Build history of the part. All positions in model axes, mm. Face numbers are marked on the shaded views. A direction names the side the tool comes from. Coordinates: 2 decimals unless noted, no trailing zeros. Order: outer loops, then holes, each group sorted by start corner. A loop starts at its lowest first (then second) coordinate and runs counter-clockwise, first axis right, second up. Notation, with made-up numbers: (7, 33.25) -> (34, 33.25) arc R18 ccw to (34, 49.25) -> close; hole circle Ø4 at (7.25, 45.5). An arc over 180 degrees is marked (long way). Write each question's results on one line, items separated by ' | '.
from build123d import *

# Parameters (mm, degrees)
PAD003_DEPTH    = 43
SKETCH004_R     = 11.5
SKETCH004_R_2   = 1.7
POCKET_DEPTH    = 4
SKETCH005_R     = 1.8
SKETCH005_W     = 20
SKETCH005_H     = 10
POCKET001_DEPTH = 3.6
CHAMFER_SIZE    = 6


with BuildPart() as part:
    # Sketch003 → Pad003 (new body)
    with BuildSketch(Plane.XY):
        Polygon((-43, 4), (-3.6, 4), (-3.6, 24), (0, 24), (0, 0), (-43, 0), align=None)
    extrude(amount=PAD003_DEPTH)

    # Sketch004 → Pocket (cut)
    with BuildSketch(Plane.XZ):
        with Locations((-21.5, 21.5)):
            Circle(SKETCH004_R)
        with Locations((-37, 37)):
            Circle(SKETCH004_R_2)
        with Locations((-6, 37)):
            Circle(SKETCH004_R_2)
        with Locations((-6, 6)):
            Circle(SKETCH004_R_2)
        with Locations((-37, 6)):
            Circle(SKETCH004_R_2)
    extrude(amount=-POCKET_DEPTH, mode=Mode.SUBTRACT)

    # Sketch005 → Pocket001 (cut)
    with BuildSketch(Plane.YZ):
        with Locations((16, 29)):
            Circle(SKETCH005_R)
        with Locations((16, 14)):
            Circle(SKETCH005_R)
        with Locations((14, 38)):
            Rectangle(SKETCH005_W, SKETCH005_H)
        with Locations((14, 5)):
            Rectangle(SKETCH005_W, SKETCH005_H)
    extrude(amount=-POCKET001_DEPTH, mode=Mode.SUBTRACT)

    # Chamfer
    chamfer_edges = [part.edges().sort_by_distance(p)[0] for p in [
        (-3.6, 4, 21.5),
    ]]
    chamfer(chamfer_edges, length=CHAMFER_SIZE)


solid = part.part
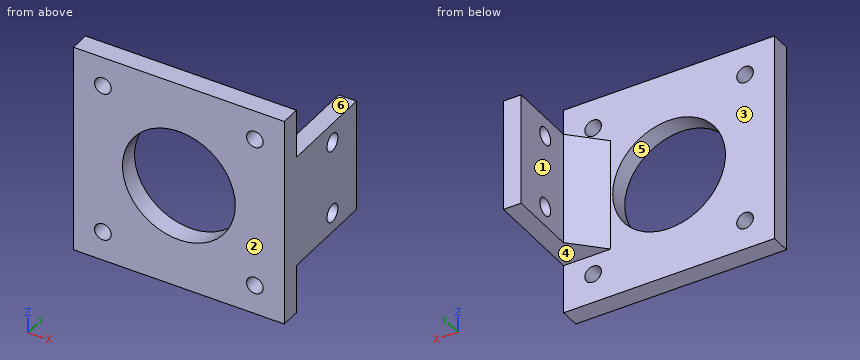
Item 1: Slice it at B-B, the plane x = -21.5. List the corners of the cut face in (y, z).
Answer:
outline: (0, 0) -> (4, 0) -> (4, 10) -> (0, 10) -> close; (0, 33) -> (4, 33) -> (4, 43) -> (0, 43) -> close
Item 2: Pin check, flat tips, straight feed: pin 1 (4.5 mm diameter, centred on x = -37, z = 6, fed in from +Y); pin 2 (11 mm diameter, centred on y = 14, z = 21.5, fed in from -X); pin 3 (2 mm diameter, centred on x = -28, z = 28.5, fed in from +Y); pin 4 (13 mm diameter, centred on x = -14, z = 24.5, fed in from +Y). Stop position of each tip, or through.
Answer:
pin 1: stops at y = 4 | pin 2: stops at x = -5.1 | pin 3: passes through | pin 4: stops at y = 6.1
Item 3: Slice it at C-C, the plane z = 37. List the corners of the cut face in (x, y), and give its area (3 significant figures).
Answer:
outline: (-43, 0) -> (-38.7, 0) -> (-38.7, 4) -> (-43, 4) -> close; (-35.3, 0) -> (-7.7, 0) -> (-7.7, 4) -> (-35.3, 4) -> close; (-4.3, 0) -> (0, 0) -> (0, 4) -> (-4.3, 4) -> close | area: 145 mm^2
Item 4: Tool access for the marked faces 1 and 2: list every direction of +Z, -Z, +X, -X, +Y, -Y with a clear straight run to the whole face (end or side of a thin tool).
Answer:
face 1: +Z, -Z, -X, +Y | face 2: +Z, -Z, +X, -X, -Y
Item 5: Slice it at D-D, the plane z = 25.5. List the corners of the cut face in (x, y).
Answer:
outline: (-43, 0) -> (-32.28, 0) -> (-32.28, 4) -> (-43, 4) -> close; (-10.72, 0) -> (0, 0) -> (0, 24) -> (-3.6, 24) -> (-3.6, 10) -> (-9.6, 4) -> (-10.72, 4) -> close
Item 6: Drill centre lines: line 1 (Z direction, x = -37, y = 2.3); line 2 (Z direction, x = -1.5, y = 16); line 3 (Z direction, x = -21.5, y = 1.25). Where is each one in solid material? Low to high. Write a range as from..to.
Answer:
line 1: z = 0..4.3, 7.7..35.3, 38.7..43 | line 2: z = 10..12.2, 15.8..27.2, 30.8..33 | line 3: z = 0..10, 33..43
Item 7: Pull direction Z, two halves, no side cores. Call the marked faces 3, 4, 5 and 6: released by +Z, released by -Z, zero draft, split by the parting line, or undercut.
Answer:
face 3: zero draft | face 4: released by -Z | face 5: undercut | face 6: released by +Z
Item 8: Slice it at A-A, the plane y = 16. List the corners of the cut face in (x, z).
Answer:
outline: (-3.6, 10) -> (0, 10) -> (0, 12.2) -> (-3.6, 12.2) -> close; (-3.6, 15.8) -> (0, 15.8) -> (0, 27.2) -> (-3.6, 27.2) -> close; (-3.6, 30.8) -> (0, 30.8) -> (0, 33) -> (-3.6, 33) -> close
